```python
from build123d import *

# Parameters (mm, degrees)
SALIENTE_EXTRUIR1_DEPTH = 125


with BuildPart() as part:
    # Croquis1 → Saliente-Extruir1 (new body)
    with BuildSketch(Plane(origin=(0, 0, 0), x_dir=(1, 0, 0), z_dir=(0, 1, 0))):
        with BuildLine():
            Line((-23, 23), (0, 23))
            Line((0, 23), (0, 0))
            Line((0, 0), (2, 0))
            Line((2, 0), (2, 24.5))
            ThreePointArc((2, 24.5), (1.853553391, 24.853553391), (1.5, 25))
            Line((1.5, 25), (-23, 25))
            Line((-23, 25), (-23, 23))
        make_face()
    extrude(amount=SALIENTE_EXTRUIR1_DEPTH)


solid = part.part
```
Can you work these out from the model? Positions are in its coordinate system, mm. A direction names the side the tool comes from. Round coordinates to 2 decimals unless told otherwise and drop trailing zeros. Loops run counter-clockwise (first coordinate to the right, second up) from the corner with the lowest first, then second, coordinate; pieces in that order, holes last. Notation, with made-up numbers: M 18,83.5 L 69,83.5 A30 ccw 69,119.5 Z; hole C 59,-36 d6. An arc over 180 degrees is marked long. Write item = value, one per line. Start each with the question number.
(1) Which directions (+Z, -Z, +X, -X, +Y, -Y) give clear straight access to the entire face, cutting with the end or side of a thin tool? Please do faces 1 (the face through (0, 62, -12)), 2 (the face through (-11, 62, -25)).
(2) Suppose I cut it at A-A on y = 37. Write out the boundary of the cut face in (x, z), plus the area to 3 significant figures.
(3) I need wall thicknesses on line 1 along X through (y, z) = (92.5, -5.5); line 2 along Z through (x, y) = (-21.5, 27.5). Which ranges of each line are inside material? Lowest first, please.
(4) Suppose I cut it at B-B on x = -3.5. Write out the boundary of the cut face in (y, z).
(5) I'm going to push flat-ended pins straight in: P1, Ø1.5, axis at y = 94.5, z = -12, coming from the -X side; P2, Ø2, axis at x = -17, y = 63, coming from the +Z side. Where does each tip first touch, or does it pass through?
(6) Suppose I cut it at C-C on z = -7. Write out the boundary of the cut face in (x, y), plus the area to 3 significant figures.
Answer block:
q1.face_1 = +Z, -X, +Y, -Y
q1.face_2 = -Z, +X, -X, +Y, -Y
q2.outline = M -23,-25 L 1.5,-25 A0.5 ccw 2,-24.5 L 2,0 L 0,0 L 0,-23 L -23,-23 Z
q2.area = 95.9 mm²
q3.line_1 = 0 to 2
q3.line_2 = -25 to -23
q4.outline = M 0,-25 L 125,-25 L 125,-23 L 0,-23 Z
q5.P1 = 0
q5.P2 = -23
q6.outline = M 0,0 L 2,0 L 2,125 L 0,125 Z
q6.area = 250 mm²
